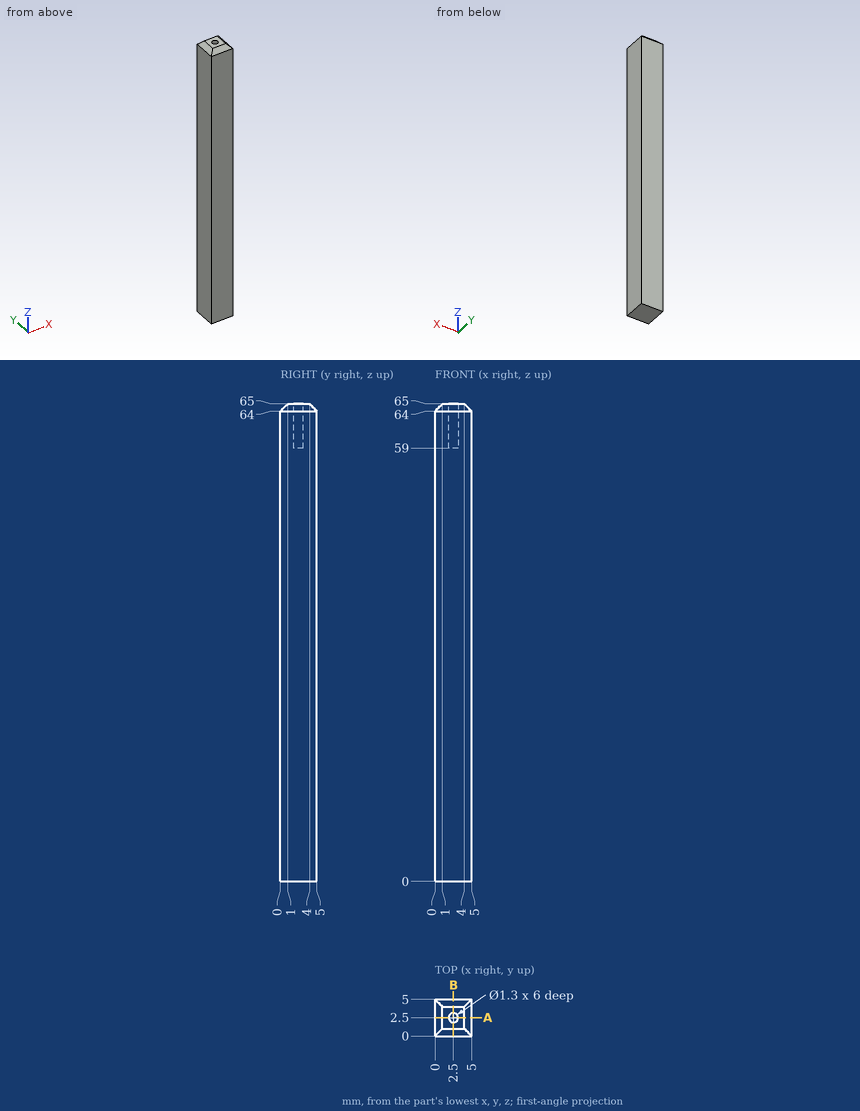
Design review of the part shown in the three views and the two pictorial views. Dimensions are in mm from the part's minimum x, y and z. Give positions to 0.01 mm unless a question says otherwise; leave off trailing zeros. Loops run counter-clockwise (first coordinate to the right, second up) from the corner with the lowest first, then second, coordinate; pieces in that order, holes last. Notation, with made-up numbers: (27.25, 5.25) -> (32.25, 5.25) arc R19 ccw to (32.25, 39.25) -> close; hole circle Ø5 at (-17.5, 85). An arc over 180 degrees is marked (long way). Answer as a JSON object with one key per item and string values. Group by question number.
Q1. Take a section at A-A (y = 2.5). Write out the cut boundary in (x, z), plus the area to 3 significant figures.
Q2. Wall thickness on line 1 along Y through (x, z) = (2.5, 61); line 2 along X through (y, z) = (2.15, 59.5); line 3 along Z through (x, y) = (4.05, 3.8): over which ranges is each line inside the solid? List them lowest first.
Q3. Insertion check: pin 1 (1 mm diameter, centred on x = 2.5, y = 2.5, fed in from +Z). The pin has a flat end and moves straight along its axis. Give the tip position at first contact, or say it passes through.
Answer below:
{
 "1": {"outline": "(0, 0) -> (5, 0) -> (5, 64) -> (4, 65) -> (3.15, 65) -> (3.15, 59) -> (1.85, 59) -> (1.85, 65) -> (1, 65) -> (0, 64) -> close", "area": "316 mm2"},
 "2": {"line 1": "y = 0 to 1.85, 3.15 to 5", "line 2": "x = 0 to 1.95, 3.05 to 5", "line 3": "z = 0 to 64.95"},
 "3": {"pin 1": "stops at z = 59"}
}
